Model file for the job. Use its own axes, mm. A direction names the side the tool comes from. Round coordinates to 2 decimals unless told otherwise and drop trailing zeros. Loops run counter-clockwise (first coordinate to the right, second up) from the corner with the lowest first, then second, coordinate; pieces in that order, holes last. Notation, with made-up numbers: M 73,42.25 L 83,42.25 A29 ccw 83,62.25 Z; hole C 59,26.5 d6. An arc over 180 degrees is marked long. Use a Markdown table: item, result. Add a question column.
Q1. Cut at B-B (y = 1.5). Give the cut face in (x, z), plus the area to 3 significant figures.
Q2. Cut at C-C (z = 0). Give the cut face in (x, y).
Q3. Probe line 1 (X direction, y = 3.4, z = 15.5); line 2 (X direction, y = 3, z = 15). List the from-to ranges inside material, lowest first. Write a range as from..to.
Q4. Mould opens along X. For faces 3 (the face through (15.34, 3.04, 14.26)), 4 (the face through (-18.7, 19.7, 18.8)), 5 (the face through (-15.45, 6.62, 15.71)), 6 (the face through (0, 20, 21)) say: +X half, -X half, draft (parallel to the pull), parting line (faces both ways), or undercut.
Q5. Cut at D-D (y = 12.5). Give the cut face in (x, z).
Q6. Tool access for faces 1 (the face through (9, 0, 9)), 2 (the face through (-18.7, 19.7, -18.8)): list every direction of +Z, -Z, +X, -X, +Y, -Y with a clear straight run to the whole face (end or side of a thin tool).
Q7. Pin check, flat tips, straight feed: pin 1 (12 mm diameter, centred on y = -15.5, z = 9, fed in from -X); pin 2 (6 mm diameter, centred on x = 6, z = 2.5, fed in from -Y); pin 3 (12 mm diameter, centred on x = 8.5, z = 15, fed in from -Y). Stop position of each tip, or through.
Q8. Cut at A-A (x = 0). Give the cut face in (y, z).
from build123d import *

# Parameters (mm, degrees)
SKETCH1_W                 = 42
SKETCH1_H                 = 42
BOSS_EXTRUDE1_DEPTH       = 40
SKETCH2_R                 = 11
BOSS_EXTRUDE2_DEPTH       = 2
SKETCH3_R                 = 2.5
BOSS_EXTRUDE3_DEPTH       = 21
CHAMFER1_SIZE             = 4.5
M3X0_5_TAPPED_HOLE2_D     = 2.5
M3X0_5_TAPPED_HOLE2_DEPTH = 6
M3X0_5_TAPPED_HOLE2_TIP   = 0.751075774


with BuildPart() as part:
    # Sketch1 → Boss-Extrude1 (new body)
    with BuildSketch(Plane(origin=(0, 0, 0), x_dir=(1, 0, 0), z_dir=(0, 1, 0))):
        Rectangle(SKETCH1_W, SKETCH1_H)
    extrude(amount=BOSS_EXTRUDE1_DEPTH)

    # Sketch2 → Boss-Extrude2 (add)
    with BuildSketch(Plane.XZ):
        Circle(SKETCH2_R)
    extrude(amount=BOSS_EXTRUDE2_DEPTH)

    # Sketch3 → Boss-Extrude3 (add)
    with BuildSketch(Plane.XZ.offset(2)):
        Circle(SKETCH3_R)
    extrude(amount=BOSS_EXTRUDE3_DEPTH)

    # Chamfer1
    chamfer1_edges = [part.edges().sort_by_distance(p)[0] for p in [
        (-21, 20, 21),
        (-21, 20, -21),
        (21, 20, -21),
        (21, 20, 21),
    ]]
    chamfer(chamfer1_edges, length=CHAMFER1_SIZE)

    # M3x0.5 Tapped Hole2
    with Locations(Plane(origin=(0, 0, 0), x_dir=(-1, 0, 0), z_dir=(0, -1, 0))):
        with Locations((15.5, 15.5), (-15.5, 15.5), (-15.5, -15.5), (15.5, -15.5)):
            Hole(M3X0_5_TAPPED_HOLE2_D / 2, depth=M3X0_5_TAPPED_HOLE2_DEPTH)
            with Locations((0, 0, -(M3X0_5_TAPPED_HOLE2_DEPTH + M3X0_5_TAPPED_HOLE2_TIP / 2))):  # 118° drill point
                Cone(0, M3X0_5_TAPPED_HOLE2_D / 2, M3X0_5_TAPPED_HOLE2_TIP, mode=Mode.SUBTRACT)


solid = part.part
Checked values:
| question | item | result |
|---|---|---|
| 1 | outline | M -21,-16.5 L -16.5,-21 L 16.5,-21 L 21,-16.5 L 21,16.5 L 16.5,21 L -16.5,21 L -21,16.5 Z; hole C -15.5,-15.5 d2.5; hole C -15.5,15.5 d2.5; hole C 15.5,-15.5 d2.5; hole C 15.5,15.5 d2.5 |
| 1 | area | 1,700 mm^2 |
| 2 | outline | M -21,0 L -11,0 L -11,-2 L -2.5,-2 L -2.5,-23 L 2.5,-23 L 2.5,-2 L 11,-2 L 11,0 L 21,0 L 21,40 L -21,40 Z |
| 3 | line 1 | x = -21..-16.75, -14.25..14.25, 16.75..21 |
| 3 | line 2 | x = -21..-16.65, -14.35..14.35, 16.65..21 |
| 4 | face 3 | undercut |
| 4 | face 4 | -X half |
| 4 | face 5 | undercut |
| 4 | face 6 | draft |
| 5 | outline | M -21,-16.5 L -16.5,-21 L 16.5,-21 L 21,-16.5 L 21,16.5 L 16.5,21 L -16.5,21 L -21,16.5 Z |
| 6 | face 1 | -Y |
| 6 | face 2 | -Z, -X, +Y, -Y |
| 7 | pin 1 | passes through |
| 7 | pin 2 | stops at y = -2 |
| 7 | pin 3 | stops at y = 0 |
| 8 | outline | M -23,-2.5 L -2,-2.5 L -2,-11 L 0,-11 L 0,-21 L 40,-21 L 40,21 L 0,21 L 0,11 L -2,11 L -2,2.5 L -23,2.5 Z |
